Source: three-view drawing plus pictorial views. Frame: mm from the lowest corner of the part. Coordinates: 2 decimals unless noted, no trailing zeros. Write each loop counter-clockwise with the first axis right and the second up, starting at its lowest first coordinate (ties: lowest second). Pieces come first, ordered by that corner, then holes. Notation, with made-up numbers: (64.25, -2.5) -> (101.25, -2.5) arc R24 cw to (101.25, 20.5) -> close; hole circle Ø6 at (-31, -38.5). An arc over 180 degrees is marked (long way). One line per item, written item: value.
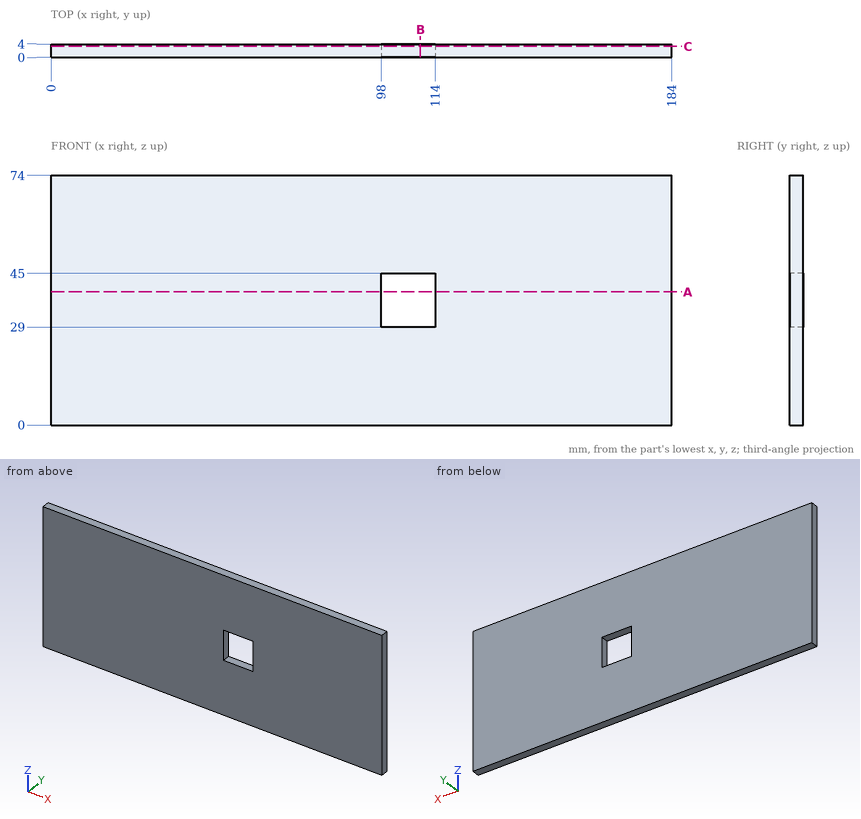
(1) Section A-A (z = 39.5). Return the cut outline in (x, y), then the cut area to 3 significant figures.
Responses:
outline: (0, 0) -> (98, 0) -> (98, 4) -> (0, 4) -> close; (114, 0) -> (184, 0) -> (184, 4) -> (114, 4) -> close
area: 672 mm2
(2) Section B-B (x = 109.5). Return the cut outline in (y, z), then the cut area to 3 significant figures.
Responses:
outline: (0, 0) -> (4, 0) -> (4, 29) -> (0, 29) -> close; (0, 45) -> (4, 45) -> (4, 74) -> (0, 74) -> close
area: 232 mm2
(3) Section C-C (y = 3.3). Return the cut outline in (x, z), then the cut area to 3 significant figures.
Responses:
outline: (0, 0) -> (184, 0) -> (184, 74) -> (0, 74) -> close; hole (98, 29) -> (114, 29) -> (114, 45) -> (98, 45) -> close
area: 13,400 mm2
(4) Line query: line 1 (Z direction, x = 111, y = 3); line 2 (X direction, y = 0.4, z = 42.5). Output: solid intervals per line, ascending. Write a range as [from, to].
Responses:
line 1: z = [0, 29], [45, 74]
line 2: x = [0, 98], [114, 184]
